Here's the drawing with two shaded views (mm, measured from the low corner). I have some questions. Round coordinates to 2 decimals unless told otherwise and drop trailing zeros. Write each loop counter-clockwise with the first axis right and the second up, starting at its lowest first coordinate (ties: lowest second). Pieces come first, ordered by that corner, then holes. Notation, with made-up numbers: M 1,-6.75 L 7,-6.75 A33 cw 7,29.25 Z; hole C 88.25,71.25 d5. An arc over 180 degrees is marked long. Answer as a JSON object with one key per item and string values. Group by question number.
1) Suppose I cut it at D-D, the plane x = 7.75. Write out the boundary of the cut face in (y, z), and give its area (3 significant figures).
2) If we mould it in two halves opening along Y, with no side actions, what happens to the marked faces 1, 2 and 3? For each: +Y half, -Y half, draft (parallel to the pull), parting line (faces both ways), or undercut.
3) Please list where these lines run through material, in increasing order: L1, parallel to Y at x = 5, z = 2; L2, parallel to X at y = 4.25, z = 2.55 (3 decimals); L3, parallel to X at y = 6, z = 1.6. Write a range as [from, to].
4) Suppose I cut it at A-A, the plane y = 5. Write out the boundary of the cut face in (x, z).
5) Suppose I cut it at C-C, the plane z = 0.95. Write out the boundary of the cut face in (x, y).
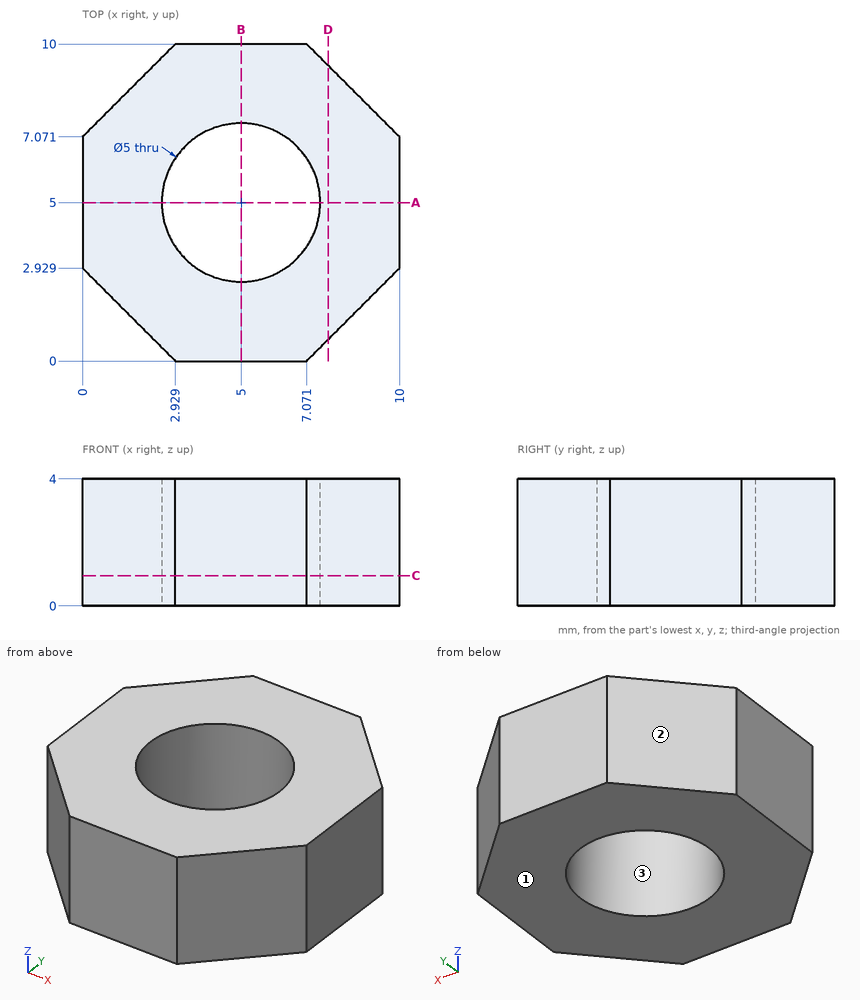
Results:
{
 "1": {"outline": "M 0.68,0 L 9.32,0 L 9.32,4 L 0.68,4 Z", "area": "34.6 mm^2"},
 "2": {"face 1": "draft", "face 2": "+Y half", "face 3": "undercut"},
 "3": {"L1": "[0, 2.5], [7.5, 10]", "L2": "[0, 2.615], [7.385, 10]", "L3": "[0, 2.71], [7.29, 10]"},
 "4": {"outline": "M 0,0 L 2.5,0 L 2.5,4 L 0,4 Z; M 7.5,0 L 10,0 L 10,4 L 7.5,4 Z"},
 "5": {"outline": "M 0,2.93 L 2.93,0 L 7.07,0 L 10,2.93 L 10,7.07 L 7.07,10 L 2.93,10 L 0,7.07 Z; hole C 5,5 d5"}
}
